Print and shaded views of the part. All mm, measured from the part's lowest x, y and z. A direction names the side the tool comes from. Give positions to 0.01 mm unless a question says otherwise; leave off trailing zeros. Loops run counter-clockwise (first coordinate to the right, second up) from the corner with the lowest first, then second, coordinate; pieces in that order, holes last. Notation, with made-up numbers: (-9, 33) -> (18, 33) arc R25 cw to (18, 46) -> close; hole circle Ø8 at (-2.5, 75). An arc over 180 degrees is marked (long way). Write each question's results on one line, items separated by ' | '. Start each with the question number.
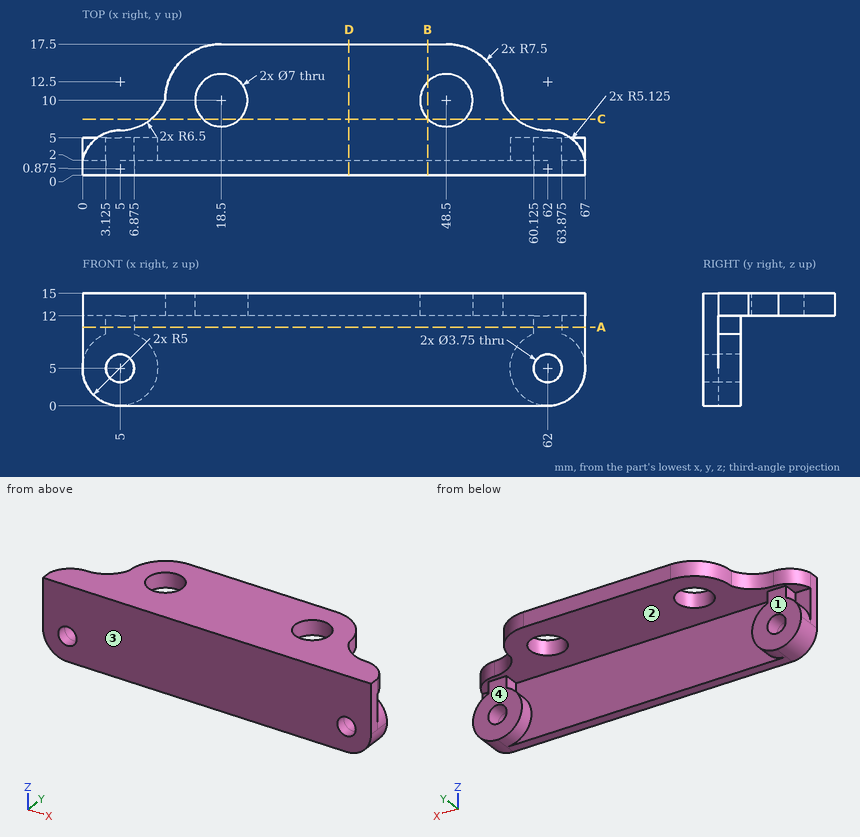
Q1. Saw through at B-B, the plane x = 46. List the corners of the cut face in (y, z), then the cut area to 3 significant figures.
Q2. Drop flat-ended pins along their axis: pin 1 (1.9 mm diameter, centred on y = 4, z = 10.5, fed in from +X); pin 2 (1.6 mm diameter, centred on x = 65, z = 8, fed in from +Y); pin 3 (2.5 mm diameter, centred on y = 4, z = 11, fed in from +X). Give the stop position or say it passes through.
Q3. Saw through at D-D, the plane x = 35.5. List the corners of the cut face in (y, z).
Q4. Mould opens along X. For the marked faces 1 and 2 say: pulls with the +X half, pulls with the -X half, needs draft (parallel to the pull), parting line crosses it, or undercut.
Q5. Saw through at A-A, the plane z = 10.5. List the corners of the cut face in (x, y) (3 decimals), then the cut area to 4 significant figures.
Q6. Wall check: L1, parallel to X at y = 4.2, z = 5 (3 decimals); L2, parallel to X at y = 1.55, z = 5 (3 decimals); L3, parallel to X at y = 9.75, z = 12.5. Give the ranges that are in metal, low to high.
Q7. Saw through at C-C, the plane y = 7.5. List the corners of the cut face in (x, z), then the cut area to 3 significant figures.
Q8. Which spindle directions (+Z, -Z, +X, -X, +Y, -Y) get a long thin tool onto all of the face, cutting with end or side? Do the marked faces 3 and 4. Say none if no direction does.
Answer block:
1) outline: (0, 0) -> (2, 0) -> (2, 12) -> (7.55, 12) -> (7.55, 15) -> (0, 15) -> close; (12.45, 12) -> (17.5, 12) -> (17.5, 15) -> (12.45, 15) -> close | area: 61.8 mm2
2) pin 1: stops at x = 64.07 | pin 2: stops at y = 5 | pin 3: stops at x = 66.54
3) outline: (0, 0) -> (2, 0) -> (2, 12) -> (17.5, 12) -> (17.5, 15) -> (0, 15) -> close
4) face 1: needs draft | face 2: undercut
5) outline: (0, 0) -> (67, 0) -> (67, 2) -> (63.875, 2) -> (63.875, 5) -> (60.125, 5) -> (60.125, 2) -> (6.875, 2) -> (6.875, 5) -> (3.125, 5) -> (3.125, 2) -> (0, 2) -> close | area: 156.5 mm2
6) L1: x = 0 to 3.125, 6.875 to 10, 57 to 60.125, 63.875 to 67 | L2: x = 0 to 3.125, 6.875 to 60.125, 63.875 to 67 | L3: x = 10.89 to 15.01, 21.99 to 45.01, 51.99 to 56.11
7) outline: (9.15, 12) -> (16.05, 12) -> (16.05, 15) -> (9.15, 15) -> close; (20.95, 12) -> (46.05, 12) -> (46.05, 15) -> (20.95, 15) -> close; (50.95, 12) -> (57.85, 12) -> (57.85, 15) -> (50.95, 15) -> close | area: 117 mm2
8) face 3: +Z, -Z, +X, -X, -Y | face 4: -Z, +X, -X, +Y
